Part model, mm, in its own coordinate system. A direction names the side the tool comes from. Give positions to 0.01 mm unless a question says otherwise; leave off trailing zeros. Write each loop counter-clockwise with the first axis right and the second up, starting at its lowest first coordinate (ties: lowest second). Pieces come first, ordered by that corner, then holes. Notation, with made-up numbers: M 89.25,64.5 L 108.25,64.5 A19 ccw 108.25,95.5 Z; hole C 69,-4 d3. An arc over 180 degrees is marked long. Use a Markdown table: item, result.
Autodesk Inventor part; units mm, degrees
ref_plane "YZ Plane" through (0, 0, 0) normal (1, 0, 0) x (0, 1, 0)
ref_plane "XZ Plane" through (0, 0, 0) normal (0, 1, 0) x (-1, 0, 0)
ref_plane "XY Plane" through (0, 0, 0) normal (0, 0, 1) x (1, 0, 0)
sketch "Эскиз1" plane through (0, 0, 0) normal (0, 0, 1) x (1, 0, 0)
  line L0 (0, 0) -> (-17, 0)
  line L1 (-17, 0) -> (-17, 7)
  line L2 (-17, 7) -> (0, 7)
  line L3 (0, 7) -> (0, 0)
  dimension "d0" = 17
  dimension "d1" = 7
extrude "Выдавливание1" add sketch "Эскиз1" along normal blind 5
sketch "Эскиз2" plane through (-17, 7, 0) normal (0, 1, 0) x (1, 0, 0)
  line L0 (17, 0) -> (0, 0)
  line L1 (0, 0) -> (0, -5)
  line L2 (17, -5) -> (0, -5)
  line L3 (17, 0) -> (17, -5)
  line L4 (17, 0) -> (0, 0)
  circle A0 centre (8.5, 0) radius 2.25
  point P0 (6.25, 0)
  point P1 (10.75, 0)
  dimension "d4" = 8.5
  dimension "d5" = 4.5
extrude "Выдавливание2" cut sketch "Эскиз2" against normal blind 100 contours A0 L0 picked at (8.074, -0.9762)
sketch "Эскиз3" plane through (-17, 7, 5) normal (0, 1, 0) x (1, 0, 0)
  arc A0 (6.25, 5) -> (10.75, 5) centre (8.5, 5) ccw
  arc A1 (5, 5) -> (12, 5) centre (8.5, 5) ccw
  arc A2 (3.5, 5) -> (13.5, 5) centre (8.5, 5) ccw
  line L0 (17, 0) -> (0, 0)
  line L1 (6.25, 5) -> (0, 5)
  line L2 (17, 5) -> (10.75, 5)
  dimension "d8" = 7
extrude "Выдавливание3" add sketch "Эскиз3" along normal blind 5 contours A1 L2 A2 L1
sketch "Эскиз5" plane through (0, 7, 5) normal (0, 1, 0) x (1, 0, 0)
  line L0 (2, 5) -> (-19, 5)
  line L1 (-19, 5) -> (-19, 0)
  line L2 (-17, -2) -> (0, -2)
  line L3 (2, 0) -> (2, 5)
  line L4 (-17, 5) -> (-17, 0)
  line L5 (0, 5) -> (0, 0)
  line L6 (0, 0) -> (-8.5, 0)
  arc A0 (-19, 0) -> (-17, -2) centre (-17, 0) ccw
  arc A1 (0, -2) -> (2, 0) centre (0, 0) ccw
  arc A2 (-13.5, 5) -> (-8.5, 0) centre (-8.5, 5) ccw
  line L7 (-13.5, 5) -> (-17, 5)
  line L8 (-17, 5) -> (-17, 0)
  line L9 (-8.5, 0) -> (-17, 0)
  arc A3 (-8.5, 0) -> (-3.5, 5) centre (-8.5, 5) ccw
  line L10 (0, 0) -> (-8.5, 0)
  line L11 (0, 5) -> (0, 0)
  line L12 (0, 5) -> (-3.5, 5)
  dimension "d11" = 2
  dimension "d12" = 2
  dimension "d13" = 2
  dimension "d14" = 2
extrude "Выдавливание4" add sketch "Эскиз5" against normal blind 1 contours L3 A1 L2 A0 L1 L0 L4 L9 L6 L5
sketch "Эскиз6" plane through (0, 0, 0) normal (0, 0, -1) x (-1, 0, 0)
  circle A0 centre (3.5, 4) radius 1
  circle A1 centre (13.5, 4) radius 1
  line L0 (8.5, 7.7891) -> (8.5, -0.9569)
  line L1 (6.25, 0) -> (0, 0)
  dimension "d17" = 2
  dimension "d18" = 2
  dimension "d19" = 10
  dimension "d20" = 5
  dimension "d21" = 4
extrude "Выдавливание5" cut sketch "Эскиз6" against normal blind 3
properties part number "держатель проводной"
1. Drop flat-ended pins along their axis: P1, Ø2.5, axis at y = 2, z = 3, coming from the +X side; P2, Ø1.5, axis at x = -17, y = 1.5, coming from the +Z side; P3, Ø1.6, axis at x = -3.5, y = 4, coming from the -Z side. Give the stop position or say it passes through.
Findings below:
| item | result |
|---|---|
| P1 | x = 0 |
| P2 | z = 5 |
| P3 | z = 3 |
2. Cut at D-D, the plane x = -8.5. Give the cut face in (y, z).
Findings below:
| item | result |
|---|---|
| outline | M 0,2.25 L 7,2.25 L 7,3.5 L 12,3.5 L 12,5 L 7,5 L 7,7 L 6,7 L 6,5 L 0,5 Z |
3. Tool access for faces 1 (the cylindrical face through (-2.763, 4.676, 1.479)), 2 (the flat face through (-17, 3, 2)), 3 (the flat face through (0, 3, 2)), 4 (the flat face through (-9, 3, 5)): list every direction of +Z, -Z, +X, -X, +Y, -Y with a clear straight run to the whole face (end or side of a thin tool).
Findings below:
| item | result |
|---|---|
| face 1 | -Z |
| face 2 | +Z, -Z, -X, -Y |
| face 3 | +Z, -Z, +X, -Y |
| face 4 | +Z, +X, -X, -Y |
4. Cut at A-A, the plane z = 2. Give the cut face in (x, y).
Findings below:
| item | result |
|---|---|
| outline | M -19,6 L -17,6 L -17,0 L -9.53,0 L -9.53,7 L -11.37,7 L -11.37,12 L -13.08,12 L -13.08,7 L -19,7 Z; M -7.47,0 L 0,0 L 0,6 L 2,6 L 2,7 L -3.92,7 L -3.92,12 L -5.63,12 L -5.63,7 L -7.47,7 Z; hole C -13.5,4 d2; hole C -3.5,4 d2 |
5. Cut at B-B, the plane y = 4. Give the cut face in (x, z), then the cut area to 3 significant figures.
Findings below:
| item | result |
|---|---|
| outline | M -17,0 L -14.5,0 L -14.5,3 L -12.5,3 L -12.5,0 L -10.75,0 A2.25 cw -6.25,0 L -4.5,0 L -4.5,3 L -2.5,3 L -2.5,0 L 0,0 L 0,5 L -17,5 Z |
| area | 65.0 mm2 |
6. Two-plate mould, pull along Y, no slides. Class faces 5 (the flat face through (-3, 4, 3)), 6 (the flat face through (-8.4, 0, 2.5)), 7 (the flat face through (-2, 5, 0)): released by +Y, released by -Y, zero draft, split by the parting line, or undercut.
Findings below:
| item | result |
|---|---|
| face 5 | undercut |
| face 6 | released by -Y |
| face 7 | zero draft |
7. Cut at C-C, the plane z = 4. Give the cut face in (x, y), then the cut area to 3 significant figures.
Findings below:
| item | result |
|---|---|
| outline | M -19,6 L -17,6 L -17,0 L 0,0 L 0,6 L 2,6 L 2,7 L -5.5,7 L -5.5,12 L -11.5,12 L -11.5,7 L -19,7 Z |
| area | 153 mm2 |
8. Drill centre lines: L1, parallel to Y at x = -13.5, z = 1.8; L2, parallel to Y at x = -11, z = 5.75; L3, parallel to Z at x = -2, y = 5. Where is each one in solid material? Low to high.
Findings below:
| item | result |
|---|---|
| L1 | 0 to 3, 5 to 7 |
| L2 | 6 to 7 |
| L3 | 0 to 5 |
